from build123d import *

# Parameters (mm, degrees)
SKETCH_1_W          = 60
SKETCH_1_H          = 80
EXTRUDE_1_DEPTH     = 5
SKETCH_2_R          = 1.5
SKETCH_2_R_2        = 9
CUT_EXTRUDE_1_DEPTH = 51.249378106
SKETCH_3_R          = 1.5
CUT_EXTRUDE_2_DEPTH = 51.249378106
SKETCH_4_R          = 3
CUT_EXTRUDE_3_DEPTH = 3
SKETCH_5_OUTSIDE_W  = 82.024
SKETCH_5_OUTSIDE_H  = 102.024
SKETCH_5_OUTSIDE_R  = 1.5
CUT_EXTRUDE_4_DEPTH = 51.249378106
SKETCH_6_R          = 12
CUT_EXTRUDE_5_DEPTH = 2


with BuildPart() as part:
    # 草图1 → 凸台-拉伸1 (new body)
    with BuildSketch(Plane(origin=(0, 0, 0), x_dir=(1, 0, 0), z_dir=(0, 1, 0))):
        Rectangle(SKETCH_1_W, SKETCH_1_H)
    extrude(amount=EXTRUDE_1_DEPTH)

    # 草图2 → 切除-拉伸1 (cut, through all)
    with BuildSketch(Plane(origin=(0, 5, 0), x_dir=(1, 0, 0), z_dir=(0, 1, 0))):
        with Locations(Location((20, 0, 0), (0, 0, 270))):
            Circle(SKETCH_2_R)
        with Locations(Location((-10, -17.320508076, 0), (0, 0, 270))):
            Circle(SKETCH_2_R)
        with Locations(Location((-10, 17.320508076, 0), (0, 0, 270))):
            Circle(SKETCH_2_R)
        with Locations(Location((0, 0, 0), (0, 0, 270))):
            Circle(SKETCH_2_R_2)
    extrude(amount=-CUT_EXTRUDE_1_DEPTH, mode=Mode.SUBTRACT)

    # 草图3 → 切除-拉伸2 (cut, through all)
    with BuildSketch(Plane(origin=(0, 5, 0), x_dir=(1, 0, 0), z_dir=(0, 1, 0))):
        with Locations(Location((-25, 30, 0), (0, 0, 270))):
            Circle(SKETCH_3_R)
        with Locations(Location((25, 30, 0), (0, 0, 270))):
            Circle(SKETCH_3_R)
        with Locations(Location((-25, -30, 0), (0, 0, 270))):
            Circle(SKETCH_3_R)
        with Locations(Location((25, -30, 0), (0, 0, 270))):
            Circle(SKETCH_3_R)
        with Locations(Location((-16, -31, 0), (0, 0, 270))):
            Circle(SKETCH_3_R)
        with Locations(Location((16, -31, 0), (0, 0, 270))):
            Circle(SKETCH_3_R)
        with Locations(Location((16, 31, 0), (0, 0, 90))):
            Circle(SKETCH_3_R)
        with Locations(Location((-16, 31, 0), (0, 0, 90))):
            Circle(SKETCH_3_R)
    extrude(amount=-CUT_EXTRUDE_2_DEPTH, mode=Mode.SUBTRACT)

    # 草图4 → 切除-拉伸3 (cut)
    with BuildSketch(Plane.XZ):
        with Locations(Location((-25, 30, 0), (0, 0, 270))):
            Circle(SKETCH_4_R)
        with Locations(Location((25, 30, 0), (0, 0, 270))):
            Circle(SKETCH_4_R)
        with Locations(Location((25, -30, 0), (0, 0, 270))):
            Circle(SKETCH_4_R)
        with Locations(Location((-25, -30, 0), (0, 0, 270))):
            Circle(SKETCH_4_R)
        with Locations(Location((-16, 31, 0), (0, 0, 270))):
            Circle(SKETCH_4_R)
        with Locations(Location((16, 31, 0), (0, 0, 270))):
            Circle(SKETCH_4_R)
        with Locations(Location((-16, -31, 0), (0, 0, 270))):
            Circle(SKETCH_4_R)
        with Locations(Location((16, -31, 0), (0, 0, 270))):
            Circle(SKETCH_4_R)
    extrude(amount=-CUT_EXTRUDE_3_DEPTH, mode=Mode.SUBTRACT)

    # 草图5 outside → 切除-拉伸4 (cut, through all)
    # profile 1 of 8: a face of its own
    with BuildSketch(Plane(origin=(0, 5, 0), x_dir=(1, 0, 0), z_dir=(0, 1, 0))):
        Rectangle(SKETCH_5_OUTSIDE_W, SKETCH_5_OUTSIDE_H)
        with BuildLine():
            Line((-20, -36), (-20, -40))
            Line((-20, -40), (20, -40))
            Line((20, -40), (20, -36))
            ThreePointArc((20, -36), (19.292893219, -34.292893219), (21, -35))
            Line((21, -35), (30, -35))
            Line((30, -35), (30, 35))
            Line((30, 35), (21, 35))
            ThreePointArc((21, 35), (19.292893219, 34.292893219), (20, 36))
            Line((20, 36), (20, 40))
            Line((20, 40), (-20, 40))
            Line((-20, 40), (-20, 36))
            ThreePointArc((-20, 36), (-19.292893219, 35.707106781), (-19, 35))
            ThreePointArc((-19, 35), (-20, 34), (-21, 35))
            Line((-21, 35), (-30, 35))
            Line((-30, 35), (-30, -35))
            Line((-30, -35), (-21, -35))
            ThreePointArc((-21, -35), (-20, -34), (-19, -35))
            ThreePointArc((-19, -35), (-19.292893219, -35.707106781), (-20, -36))
        make_face(mode=Mode.SUBTRACT)
    # profile 2 of 8: a face of its own
    with BuildSketch(Plane(origin=(0, 5, 0), x_dir=(1, 0, 0), z_dir=(0, 1, 0))):
        with Locations(Location((-25, -30, 0), (0, 0, 270))):
            Circle(SKETCH_5_OUTSIDE_R)
    # profile 3 of 8: a face of its own
    with BuildSketch(Plane(origin=(0, 5, 0), x_dir=(1, 0, 0), z_dir=(0, 1, 0))):
        with Locations(Location((-10, -17.320508076, 0), (0, 0, 270))):
            Circle(SKETCH_5_OUTSIDE_R)
    # profile 4 of 8: a face of its own
    with BuildSketch(Plane(origin=(0, 5, 0), x_dir=(1, 0, 0), z_dir=(0, 1, 0))):
        with Locations(Location((25, -30, 0), (0, 0, 270))):
            Circle(SKETCH_5_OUTSIDE_R)
    # profile 5 of 8: a face of its own
    with BuildSketch(Plane(origin=(0, 5, 0), x_dir=(1, 0, 0), z_dir=(0, 1, 0))):
        with Locations(Location((20, 0, 0), (0, 0, 270))):
            Circle(SKETCH_5_OUTSIDE_R)
    # profile 6 of 8: a face of its own
    with BuildSketch(Plane(origin=(0, 5, 0), x_dir=(1, 0, 0), z_dir=(0, 1, 0))):
        with Locations(Location((-10, 17.320508076, 0), (0, 0, 270))):
            Circle(SKETCH_5_OUTSIDE_R)
    # profile 7 of 8: a face of its own
    with BuildSketch(Plane(origin=(0, 5, 0), x_dir=(1, 0, 0), z_dir=(0, 1, 0))):
        with Locations(Location((-25, 30, 0), (0, 0, 270))):
            Circle(SKETCH_5_OUTSIDE_R)
    # profile 8 of 8: a face of its own
    with BuildSketch(Plane(origin=(0, 5, 0), x_dir=(1, 0, 0), z_dir=(0, 1, 0))):
        with Locations(Location((25, 30, 0), (0, 0, 270))):
            Circle(SKETCH_5_OUTSIDE_R)
    extrude(amount=-CUT_EXTRUDE_4_DEPTH, mode=Mode.SUBTRACT)

    # 草图6 → 切除-拉伸5 (cut)
    with BuildSketch(Plane.XZ):
        with Locations(Location((0, 0, 0), (0, 0, 270))):
            Circle(SKETCH_6_R)
    extrude(amount=-CUT_EXTRUDE_5_DEPTH, mode=Mode.SUBTRACT)


solid = part.part
Can you work these out from the model? Positions are in its coordinate system, mm. A direction names the side the tool comes from. Round coordinates to 2 decimals unless told otherwise and drop trailing zeros. Order: outer loops, then holes, each group sorted by start corner. A loop starts at its lowest first (then second) coordinate and runs counter-clockwise, first axis right, second up. Notation, with made-up numbers: (-6.75, 7.25) -> (0.25, 7.25) arc R20 ccw to (0.25, 23.25) -> close; hole circle Ø7 at (-30.5, 32.25). An arc over 180 degrees is marked (long way). Write each question's results on one line, items separated by ' | '. Start each with the question number.
Item 1: If we section it at C-C, the plane z = -6.5: Write out the boundary of the cut face in (x, y), then the cut area to 3 significant figures.
Item 2: Thinking about a two-plate mould opening in Z: for faces 1 (the cylindrical face through (-17.8, 1.5, -28.6)), 2 (the flat face through (30, 2, 0)), 3 (the flat face through (-25, 3, -35)), which applies, +Z half, -Z half, draft (parallel to the pull), parting line (faces both ways), or undercut?
Item 3: If we section it at B-B, the plane x = 0: Write out the boundary of the cut face in (y, z).
Item 4: Will these pins go through, and if not, where does the flat tip stop? pin 1 (2.5 mm diameter, centred on x = -10, z = -17.32, fed in from +Y); pin 2 (5.5 mm diameter, centred on x = -25, z = 30, fed in from -Y); pin 3 (1.2 mm diameter, centred on y = 3.5, z = -37.5, fed in from +X); pin 4 (2.5 mm diameter, centred on x = 24, y = 2, fed in from +Z).
Item 5: Please list where these lines run through material, in increasing order: L1, parallel to X at y = 0.2, z = -30.5; L2, parallel to X at y = 2.25, z = -30; L3, parallel to Z at x = 14, y = 2.95.
Item 6: If we section it at D-D, the plane x = -25: Write out the boundary of the cut face in (y, z).
Item 7: Which directions (+Z, -Z, +X, -X, +Y, -Y) give clear straight access to the entire face, cutting with the end or side of a thin tool? Please do faces 4 (the flat face through (9, 2, -2)), 5 (the cylindrical face through (26.01, 4.01, 28.89)).
Item 8: If we section it at A-A, the plane x = 16: Write out the boundary of the cut face in (y, z), then the cut area to 3 significant figures.
Results:
1) outline: (-30, 0) -> (-10.09, 0) -> (-10.09, 2) -> (-6.22, 2) -> (-6.22, 5) -> (-30, 5) -> close; (6.22, 2) -> (10.09, 2) -> (10.09, 0) -> (30, 0) -> (30, 5) -> (6.22, 5) -> close | area: 222 mm2
2) face 1: undercut | face 2: draft | face 3: -Z half
3) outline: (0, -40) -> (5, -40) -> (5, -9) -> (2, -9) -> (2, -12) -> (0, -12) -> close; (0, 12) -> (2, 12) -> (2, 9) -> (5, 9) -> (5, 40) -> (0, 40) -> close
4) pin 1: passes through | pin 2: stops at y = 3 | pin 3: stops at x = 20 | pin 4: stops at z = 35
5) L1: x = -30 to -27.96, -22.04 to -18.96, -13.04 to 13.04, 18.96 to 22.04, 27.96 to 30 | L2: x = -30 to -28, -22 to -18.83, -13.17 to 13.17, 18.83 to 22, 28 to 30 | L3: z = -40 to -33.24, -28.76 to 28.76, 33.24 to 40
6) outline: (0, -35) -> (5, -35) -> (5, -31.5) -> (3, -31.5) -> (3, -33) -> (0, -33) -> close; (0, -27) -> (3, -27) -> (3, -28.5) -> (5, -28.5) -> (5, 28.5) -> (3, 28.5) -> (3, 27) -> (0, 27) -> close; (0, 33) -> (3, 33) -> (3, 31.5) -> (5, 31.5) -> (5, 35) -> (0, 35) -> close
7) face 4: -Y | face 5: +Y, -Y
8) outline: (0, -40) -> (5, -40) -> (5, -32.5) -> (3, -32.5) -> (3, -34) -> (0, -34) -> close; (0, -28) -> (3, -28) -> (3, -29.5) -> (5, -29.5) -> (5, 29.5) -> (3, 29.5) -> (3, 28) -> (0, 28) -> close; (0, 34) -> (3, 34) -> (3, 32.5) -> (5, 32.5) -> (5, 40) -> (0, 40) -> close | area: 352 mm2
